Build history of the part. All positions in model axes, mm. Face numbers are marked on the shaded views. Give positions to 0.01 mm unless a question says otherwise; leave off trailing zeros. Write each loop counter-clockwise with the first axis right and the second up, starting at its lowest first coordinate (ties: lowest second). Pieces come first, ordered by that corner, then holes. Notation, with made-up numbers: (75.25, 24) -> (83.25, 24) arc R14 cw to (83.25, 46) -> close; hole circle Ø8 at (-21.5, 9). An arc over 180 degrees is marked (long way). Write item = value, one per line. Start each with the question number.
Q1. Saw through at C-C, the plane z = 4. List the corners of the cut face in (x, y), then the cut area to 3 significant figures.
Q2. Drop flat-ended pins along their axis: P1, Ø2, axis at x = -37, y = 68.68, coming from the -Z side; P2, Ø4, axis at x = -163, y = 68.68, coming from the -Z side. Give the stop position or say it passes through.
Q3. Wall check: line 1 (Y direction, x = -163, z = 9.2); line 2 (Y direction, x = -128.5, z = 1); line 3 (X direction, y = 131.5, z = 4.5). Give the ranges that are in metal, low to high.
Q4. Mould opens along Y. For the marked faces 1 and 2 say: pulls with the +Y half, pulls with the -Y half, needs draft (parallel to the pull), parting line crosses it, or undercut.
Q5. Saw through at B-B, the plane y = 65. List the corners of the cut face in (x, z), then the cut area to 3 significant figures.
Q6. Saw through at A-A, the plane x = -94.5. List the corners of the cut face in (y, z), then the cut area to 3 significant figures.
Q7. Saw through at D-D, the plane x = -33. List the corners of the cut face in (y, z), then the cut area to 3 significant figures.
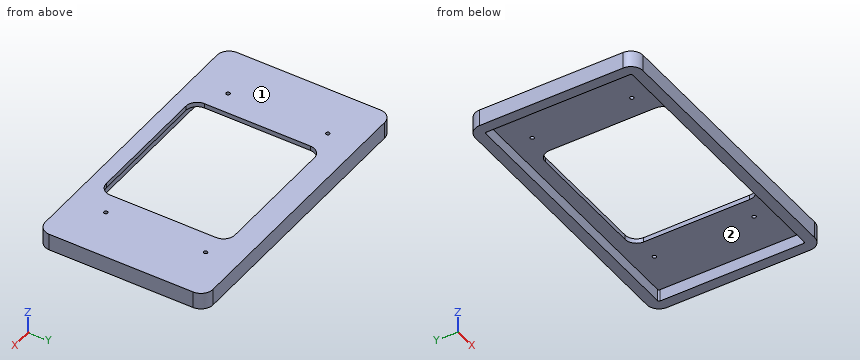
Autodesk Inventor part; units mm, degrees
ref_plane "Work Plane6" through (-196, 0, 0) normal (0, 0, -1) x (-1, 0, 0)
ref_plane "Work Plane3" through (-196, 0, 0) normal (0, 0, -1) x (-1, 0, 0)
ref_plane "Work Plane2" through (-196, 0, 10) normal (0, 0, 1) x (1, 0, 0)
ref_plane "Work Plane5" through (-196, 0, 0) normal (0, 0, 1) x (1, 0, 0)
sketch "Sketch13" plane through (-196, 0, 0) normal (0, 0, 1) x (1, 0, 0)
  line L0 (7.5, 44.9846) -> (184.5156, 44.9846)
  line L1 (192.5, 52.4846) -> (192.5, 147.9846)
  line L2 (184.5, 155.9846) -> (7.5, 155.9846)
  line L3 (-0.5, 147.9846) -> (-0.5, 52.9846)
  arc A0 (-0.5, 52.9846) -> (7.5, 44.9846) centre (7.5, 52.9846) ccw
  arc A1 (184.5156, 44.9846) -> (192.5, 52.4846) centre (184.5156, 52.9846) ccw
  arc A2 (7.5, 155.9846) -> (-0.5, 147.9846) centre (7.5, 147.9846) ccw
  arc A3 (192.5, 147.9846) -> (184.5, 155.9846) centre (184.5, 147.9846) ccw
  line L4 (6.5, 147.9846) -> (6.5, 52.9846)
  arc A4 (6.5, 52.9846) -> (7.5, 51.9846) centre (7.5, 52.9846) ccw
  line L5 (7.5, 51.9846) -> (184.5156, 51.9846)
  arc A5 (184.5156, 51.9846) -> (185.5, 52.8084) centre (184.5156, 52.9846) ccw
  line L6 (185.5, 52.8084) -> (185.5, 147.9846)
  arc A6 (185.5, 147.9846) -> (184.5, 148.9846) centre (184.5, 147.9846) ccw
  line L7 (184.5, 148.9846) -> (7.5, 148.9846)
  arc A7 (7.5, 148.9846) -> (6.5, 147.9846) centre (7.5, 147.9846) ccw
  point P0 (-0.5, 44.9846)
  point P1 (192.5, 155.9846)
  point P2 (192.5, 44.9846)
  point P3 (-0.5, 155.9846)
  dimension "d79" = 8
  dimension "d112" = 8
  dimension "d117" = 7
extrude "Extrusion9" add sketch "Sketch13" along normal blind 11.1
ref_plane "Work Plane6" through (-196, 0, 0) normal (0, 0, -1) x (-1, 0, 0)
sketch "Sketch14" plane through (-196, 0, 0) normal (0, 0, -1) x (-1, 0, 0)
  line L0 (-144.7002, 132.1649) -> (-144.7002, 67.5846)
  line L1 (-47.7002, 67.5846) -> (-47.7002, 132.5846)
  line L2 (-55.2002, 140.0846) -> (-137.2002, 140.0846)
  line L3 (-144.7002, 132.5846) -> (-144.7002, 132.1649)
  arc A0 (-137.2002, 140.0846) -> (-144.7002, 132.5846) centre (-137.2002, 132.5846) ccw
  arc A1 (-47.7002, 132.5846) -> (-55.2002, 140.0846) centre (-55.2002, 132.5846) ccw
  line L4 (-192.5, 100.2346) -> (-248.457, 100.2346)
  line L5 (-96, 155.9846) -> (-96, 209.6502)
  line L6 (-47.7002, 67.5846) -> (-47.7002, 62.4846)
  line L7 (-144.7002, 67.5846) -> (-144.7002, 62.4846)
  line L8 (-137.2002, 54.9846) -> (-55.2002, 54.9846)
  arc A2 (-55.2002, 54.9846) -> (-47.7002, 62.4846) centre (-55.2002, 62.4846) ccw
  arc A3 (-144.7002, 62.4846) -> (-137.2002, 54.9846) centre (-137.2002, 62.4846) ccw
  line L9 (-184.5, 155.9846) -> (-7.5, 155.9846)
  line L10 (-192.5, 52.4846) -> (-192.5, 147.9846)
  line L11 (0.5, 147.9846) -> (0.5, 52.9846)
  line L12 (0.5, 147.9846) -> (0.5, 163.3157)
  line L13 (0.5, 163.3157) -> (-33.72, 163.3157)
  circle A4 centre (-159, 134.6846) radius 1.25
  line L14 (-159, 134.6846) -> (-159, 68.6846)
  circle A5 centre (-159, 68.6846) radius 1.25
  line L15 (-159, 68.6846) -> (-33, 68.6846)
  circle A6 centre (-33, 68.6846) radius 1.25
  line L16 (-33, 68.6846) -> (-33, 134.6846)
  circle A7 centre (-33, 134.6846) radius 1.25
  line L17 (-184.5156, 51.9846) -> (-7.5, 51.9846)
  point P0 (-196, 0)
  point P1 (-181.3, 148.9846)
  point P2 (-13.3, 148.9846)
  point P3 (-47.7002, 140.0846)
  point P4 (-144.7002, 140.0846)
  dimension "d80" = 97
  dimension "d83" = 7.5
  dimension "d111" = 7.5
  dimension "d126" = 34.22
  dimension "d132" = 2.5
  dimension "d133" = 33.5
  dimension "d134" = 21.3
  dimension "d135" = 66
  dimension "d136" = 2.5
  dimension "d138" = 126
  dimension "d139" = 2.5
  dimension "d140" = 2.5
  dimension "d142" = 3
ref_plane "Work Plane3" through (-196, 0, 0) normal (0, 0, -1) x (-1, 0, 0)
sketch "Sketch16" plane through (-196, 0, 0) normal (0, 0, -1) x (-1, 0, 0)
  line L0 (-181.3, 148.9846) -> (-6.5, 148.9846)
  line L1 (-6.5, 148.9846) -> (-6.5, 47)
  line L2 (-6.5, 47) -> (-181.3, 47)
  line L3 (-6.5, 52.9846) -> (-6.5, 147.9846)
  line L4 (-185.5, 147.9846) -> (-185.5, 52.8084)
  line L5 (-181.3, 47) -> (-185.5, 47)
  line L6 (-185.5, 47) -> (-185.5, 148.9846)
  line L7 (-185.5, 148.9846) -> (-6.5, 148.9846)
  line L8 (-6.5, 148.9846) -> (-185.5, 148.9846)
  point P0 (-196, 0)
extrude "Extrusion11" add sketch "Sketch16" against normal up to surface (11.1 mm away)
extrude "Extrusion12" cut sketch "Sketch14" against normal up to surface (11.1 mm away)
ref_plane "Work Plane2" through (-196, 0, 10) normal (0, 0, 1) x (1, 0, 0)
sketch "Sketch18" plane through (-196, 0, 10) normal (0, 0, 1) x (1, 0, 0)
  point P0 (196, 0)
extrude "Extrusion14" cut sketch "Sketch13" along normal blind 8 contours A7 L7 A6 L6 A5 L5 A4 L4
properties part number "Ventilator Screen Arm 01" material "PAEK Plastic"
Report:
q1.outline = (-196.5, 52.98) arc R8 ccw to (-188.5, 44.98) -> (-11.48, 44.98) arc R8 ccw to (-3.5, 52.48) -> (-3.5, 147.98) arc R8 ccw to (-11.5, 155.98) -> (-188.5, 155.98) arc R8 ccw to (-196.5, 147.98) -> close; hole (-189.5, 52.98) arc R1 ccw to (-188.5, 51.98) -> (-11.48, 51.98) arc R1 ccw to (-10.5, 52.81) -> (-10.5, 147.98) arc R1 ccw to (-11.5, 148.98) -> (-188.5, 148.98) arc R1 ccw to (-189.5, 147.98) -> close
q1.area = 4,010 mm2
q2.P1 = through
q2.P2 = 8
q3.line_1 = 44.98 to 67.43, 69.93 to 133.43, 135.93 to 155.98
q3.line_2 = 44.98 to 51.98, 148.98 to 155.98
q3.line_3 = -196.5 to -189.5, -10.5 to -3.5
q4.face_1 = needs draft
q4.face_2 = undercut
q5.outline = (-196.5, 0) -> (-189.5, 0) -> (-189.5, 8) -> (-148.3, 8) -> (-148.3, 11.1) -> (-196.5, 11.1) -> close; (-51.3, 8) -> (-10.5, 8) -> (-10.5, 0) -> (-3.5, 0) -> (-3.5, 11.1) -> (-51.3, 11.1) -> close
q5.area = 410 mm2
q6.outline = (44.98, 0) -> (51.98, 0) -> (51.98, 8) -> (54.98, 8) -> (54.98, 11.1) -> (44.98, 11.1) -> close; (140.08, 8) -> (148.98, 8) -> (148.98, 0) -> (155.98, 0) -> (155.98, 11.1) -> (140.08, 11.1) -> close
q6.area = 192 mm2
q7.outline = (44.98, 0) -> (51.98, 0) -> (51.98, 8) -> (148.98, 8) -> (148.98, 0) -> (155.98, 0) -> (155.98, 11.1) -> (44.98, 11.1) -> close
q7.area = 456 mm2
